```python
from build123d import *

# Parameters (mm, degrees)
SKETCH_1_R      = 2.6
SKETCH_1_R_2    = 1.6
EXTRUDE_1_DEPTH = 9


with BuildPart() as part:
    # 草图1 → 凸台-拉伸1 (new body)
    with BuildSketch(Plane(origin=(0, 0, 0), x_dir=(1, 0, 0), z_dir=(0, 1, 0))):
        with Locations(Location((0, 0, 0), (0, 0, 270))):
            Circle(SKETCH_1_R)
        with Locations(Location((0, 0, 0), (0, 0, 270))):
            Circle(SKETCH_1_R_2, mode=Mode.SUBTRACT)
    extrude(amount=EXTRUDE_1_DEPTH)

    # 草图2 → 切除-旋转1 (revolve, cut)
    with BuildSketch(Plane.XY, mode=Mode.PRIVATE) as cut_revolve_1_sk:
        Polygon((-2.6, 5.366025404), (-2.1, 4.5), (-2.6, 3.633974596), align=None)
    revolve(cut_revolve_1_sk.sketch.rotate(Axis((0, 9, 0), (0, -1, 0)), 270), axis=Axis((0, 9, 0), (0, -1, 0)), mode=Mode.SUBTRACT)


solid = part.part
```
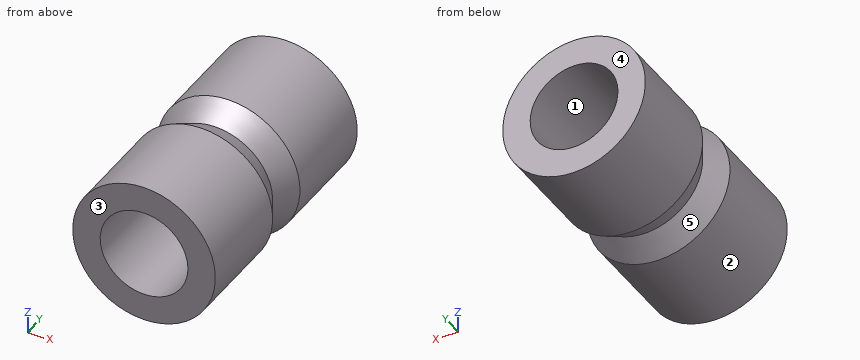
Input: part model. Units: mm. Frame: model coordinates. Face numbers are marked on the shaded views. A direction names the side the tool comes from. Give positions to 0.01 mm unless a question says otherwise; leave off trailing zeros. Loops run counter-clockwise (first coordinate to the right, second up) from the corner with the lowest first, then second, coordinate; pieces in that order, holes last. Notation, with made-up numbers: M 75,82 L 100,82 A25 cw 100,106 Z; hole C 58,53 d2. An arc over 180 degrees is marked long. Answer as CSV lines item,"result". Start each with the question number.
1. Pull-direction query (X, two-part tool) for the marked faces 1, 2 and 3; classes: released by +X, released by -X, zero draft, split by the parting line, or undercut.
2. Section A-A on z = 0. Return loops of the section in (x, y), plus the area to 3 significant figures.
3. Section C-C on y = 0.5. Return loops of the section in (x, z), plus the area to 3 significant figures.
4. Line query: L1, parallel to X at y = 6, z = 0; L2, parallel to Y at x = 1.3, z = -2.15; L3, parallel to X at y = 3.5, z = -1.3. Output: solid intervals per line, ascending.
5. Reachability of the marked faces 4 and 5 from +Z, -Z, +X, -X, +Y, -Y: full face, straight path, thin tool, end or side. Return the list, or none.
6. Section B-B on x = 0. Return loops of the section in (y, z).
Computed values:
1,face 1,"undercut"
1,face 2,"split by the parting line"
1,face 3,"zero draft"
2,outline,"M -2.6,0 L -1.6,0 L -1.6,9 L -2.6,9 L -2.6,5.37 L -2.1,4.5 L -2.6,3.63 Z; M 1.6,0 L 2.6,0 L 2.6,3.63 L 2.1,4.5 L 2.6,5.37 L 2.6,9 L 1.6,9 Z"
2,area,"17.1 mm²"
3,outline,"C 0,0 d5.2; hole C 0,0 d3.2"
3,area,"13.2 mm²"
4,L1,"x = -2.6 to -1.6, 1.6 to 2.6"
4,L2,"y = 0 to 3.79, 5.21 to 9"
4,L3,"x = -2.25 to -0.93, 0.93 to 2.25"
5,face 4,"+Z, -Z, +X, -X, +Y"
5,face 5,"none"
6,outline,"M 0,-2.6 L 3.63,-2.6 L 4.5,-2.1 L 5.37,-2.6 L 9,-2.6 L 9,-1.6 L 0,-1.6 Z; M 0,1.6 L 9,1.6 L 9,2.6 L 5.37,2.6 L 4.5,2.1 L 3.63,2.6 L 0,2.6 Z"
